from build123d import *

# Parameters (mm, degrees)
F1_W     = 44.45
F1_H     = 12.699974
F2_DEPTH = 12.7
F3_R     = 0.381
F3_R_2   = 0.403108
F4_DEPTH = 12.701
F5_W     = 2.54
F5_H     = 2.54
F6_DEPTH = 12.7
F7_W     = 6.35
F7_H     = 1.27
F7_H_2   = 3.81
F7_W_2   = 1.27
F7_H_3   = 6.35
F7_H_4   = 5.08
F8_DEPTH = 1.016


with BuildPart() as f2:
    # F1 (on face) → F2 (new body)
    with BuildSketch(Plane.XY):
        with Locations((0, 0.168821)):
            Rectangle(F1_W, F1_H)
    extrude(amount=F2_DEPTH)

    # F3 (on face) → F4 (cut, through all)
    with BuildSketch(Plane.XY.offset(12.7)):
        with Locations((-18.92253, -5.355717)):
            Circle(F3_R)
        with Locations((-19.303555, -3.895014)):
            Circle(F3_R)
        with Locations((-17.398416, -1.608836)):
            Circle(F3_R)
        with Locations((-18.92253, 1.883105)):
            Circle(F3_R_2)
        with Locations((-19.049302, 3.915029)):
            Circle(F3_R)
        with Locations((-19.176098, 5.630012)):
            Circle(F3_R)
        with Locations((-9.079903, 3.915029)):
            Circle(F3_R)
        with Locations((-7.746632, 1.184453)):
            Circle(F3_R)
        with Locations((-8.762251, -3.132963)):
            Circle(F3_R)
        with Locations((-5.917971, -3.972179)):
            Circle(F3_R)
        with Locations((-4.190606, -0.656615)):
            Circle(F3_R)
        with Locations((-2.984132, 1.121054)):
            Circle(F3_R)
        with Locations((-5.523878, 4.422826)):
            Circle(F3_R)
        with Locations((0.064084, 0.042037)):
            Circle(F3_R)
        with Locations((1.90514, 2.136673)):
            Circle(F3_R)
        with Locations((3.988689, 0.193624)):
            Circle(F3_R)
        with Locations((8.382508, -5.165547)):
            Circle(F3_R)
        with Locations((5.906389, 3.979088)):
            Circle(F3_R)
        with Locations((4.127881, 5.503215)):
            Circle(F3_R)
        with Locations((11.557508, 4.994732)):
            Circle(F3_R)
        with Locations((16.256635, 4.867961)):
            Circle(F3_R)
        with Locations((15.748381, -4.912004)):
            Circle(F3_R)
    extrude(amount=-F4_DEPTH, mode=Mode.SUBTRACT)

    # F5 (on face) → F6 (join, through all)
    with BuildSketch(Plane.XY.offset(12.7)):
        with Locations((-1.27, 7.788808)):
            Rectangle(F5_W, F5_H)
    extrude(amount=-F6_DEPTH)

    # F7 (on face) → F8 (join)
    with BuildSketch(Plane.XY.offset(12.7)):
        with Locations((-0.919895, 5.883808)):
            Rectangle(F7_W, F7_H)
        with Locations((-0.996524, -4.276166)):
            Rectangle(F7_W, F7_H_2)
        with Locations((21.59, 0.039154)):
            Rectangle(F7_W_2, F7_H_3)
        with Locations((-21.59, 0.329979)):
            Rectangle(F7_W_2, F7_H_4)
    extrude(amount=F8_DEPTH)


solid = f2.part
Geometry check sheet. Reference: the model listing, model coordinates, mm. A direction names the side the tool comes from. Coordinates: 2 decimals unless noted, no trailing zeros. Write each loop counter-clockwise with the first axis right and the second up, starting at its lowest first coordinate (ties: lowest second). Pieces come first, ordered by that corner, then holes. Notation, with made-up numbers: (-20.5, -10.75) -> (-9.5, -10.75) arc R12 cw to (-9.5, -5.75) -> close; hole circle Ø3 at (66, 26.5). An arc over 180 degrees is marked (long way). One line per question, with ' | ' between items.
1. Set-up check for faces 1 (the flat face through (-1, 5.249, 13)), 2 (the flat face through (-2.54, 8, 6)), 3 (the flat face through (-22, -2.21, 13)): record each of +Z, -Z, +X, -X, +Y, -Y from which the full face is reachable in a straight line by a thin tool's end or side.
Answers:
face 1: +Z, +X, -X | face 2: +Z, -Z, -X, +Y | face 3: +Z, -X, -Y
2. Cross-section at B-B on x = 3. Record the cut outline in (y, z), and give its area (3 significant figures).
Answers:
outline: (-6.18, 0) -> (6.52, 0) -> (6.52, 12.7) -> (-6.18, 12.7) -> close | area: 161 mm²
3. Draft check along X on faces 4 (the flat face through (-20.955, 0, 13)), 5 (the flat face through (0, 8, 6)), 6 (the flat face through (22, 3.214, 13)). Enter one of: +X half, -X half, draft (parallel to the pull), parting line (faces both ways), or undercut.
Answers:
face 4: undercut | face 5: +X half | face 6: draft
4. Thickness scan on probe 1 along Y at (x, z) = (-19.5, 12); probe 2 along Z at (x, y) = (18.5, 3.5); probe 3 along Y at (x, z) = (11.5, 10). Record the ranges inside material, lowest first. Write a range as from..to.
Answers:
probe 1: y = -6.18..-4.22, -3.57..5.43, 5.83..6.52 | probe 2: z = 0..12.7 | probe 3: y = -6.18..4.62, 5.37..6.52
5. Cross-section at A-A on z = 1. State how many separate pieces and enclosed holes the cut face has, and give its area (3 significant figures).
Answers:
separate pieces: 1 | enclosed holes: 22 | area: 561 mm²
6. Depth check by flat-ended pin: pin 1 Ø0.8 at (y, z) = (7.5, 4) entering from -X; pin 2 Ø1.1 at (x, z) = (-21.5, 13.5) entering from +Y; pin 3 Ø3 at (x, y) = (11.5, -2.5) entering from +Z. Enter the tip coordinate at first touch or a pass-through.
Answers:
pin 1: stops at x = -2.54 | pin 2: stops at y = 2.87 | pin 3: stops at z = 12.7
